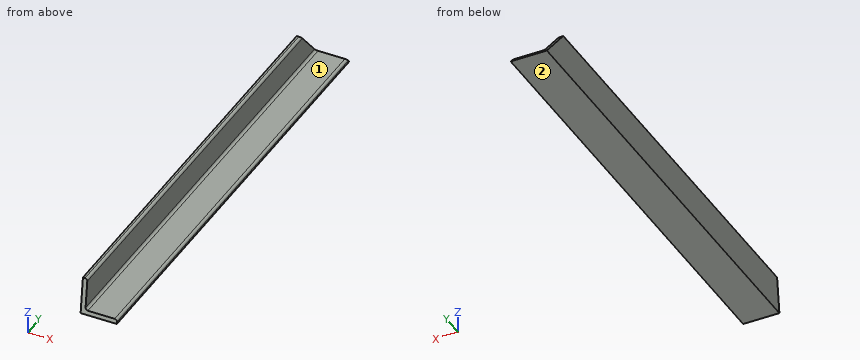
from build123d import *

# Parameters (mm, degrees)
F1_DEPTH = 474.6625
F2_R     = 5.08
F4_DEPTH = 76.2
F5_DEPTH = 76.2


with BuildPart() as f1:
    # F0 (on Front) → F1 (new body, symmetric)
    with BuildSketch(Plane.XZ):
        Polygon((0, 76.2), (0, 0), (76.2, 0), (76.2, 9.525), (9.525, 9.525), (9.525, 76.2), align=None)
    extrude(amount=F1_DEPTH, both=True)

    # F2
    f2_edges = [f1.edges().sort_by_distance(p)[0] for p in [
        (9.525, 0, 76.2),
        (9.525, 0, 9.525),
        (76.2, 0, 9.525),
    ]]
    fillet(f2_edges, radius=F2_R)

    # F3 (on face) → F4 (cut)
    with BuildSketch(Plane(origin=(0, 0, 0), x_dir=(0, -1, 0), z_dir=(-1, 0, 0))):
        Polygon((-474.6625, 76.2), (-474.6625, 0), (-407.483163, 76.2), align=None)
        Polygon((465.306316, 76.2), (474.6625, 0), (474.6625, 76.2), align=None)
    extrude(amount=-F4_DEPTH, mode=Mode.SUBTRACT)

    # F3 (on face) → F5 (cut)
    with BuildSketch(Plane(origin=(0, 0, 0), x_dir=(0, -1, 0), z_dir=(-1, 0, 0))):
        Polygon((-474.6625, 76.2), (-474.6625, 0), (-407.483163, 76.2), align=None)
        Polygon((465.306316, 76.2), (474.6625, 0), (474.6625, 76.2), align=None)
    extrude(amount=-F5_DEPTH, mode=Mode.SUBTRACT)


solid = f1.part
Check sheet for the modelled part. Datum: model origin and axes. Units: mm. Face numbers are marked on the shaded views. A direction names the side the tool comes from. Round coordinates to 2 decimals unless told otherwise and drop trailing zeros. Order: outer loops, then holes, each group sorted by start corner. A loop starts at its lowest first (then second) coordinate and runs counter-clockwise, first axis right, second up.
(1) Access from +Z, -Z, +X, -X, +Y, -Y to the whole of each face (thin tool, end or side, straight path). Record for the marked faces 1 and 2.
(2) Go/stop test with flat-tipped pins: P1, Ø2, axis at y = 212.5, z = 18, coming from the +X side (3 decimals); P2, Ø8, axis at x = 16.5, y = 344, coming from the +Z side; P3, Ø6, axis at y = 170, z = 10, coming from the +X side. Record where each tip stops, or that it passes through.
(3) Scan lines: probe 1 along X at (y, z) = (45, 67) (3 decimals); probe 2 along X at (y, z) = (-142, 5.5). Record each from-to range of solid material in increasing order.
(4) Cross-section at C-C, the plane z = 37. Enter the section's corners in (x, y) (3 decimals), and give its area (3 significant figures).
(5) Cross-section at B-B, the plane x = 24. Enter the section's corners in (y, z) (1 decimal).
(6) Cross-section at A-A, the plane y = -128. Enter the section's corners in (x, z) (3 decimals).
Check sheet entries:
1. face 1: +Z, +X, +Y, -Y
1. face 2: -Z, +X, -X, +Y, -Y
2. P1: stops at x = 9.525
2. P2: stops at z = 9.98
2. P3: stops at x = 75.51
3. probe 1: x = 0 to 9.525
3. probe 2: x = 0 to 76.09
4. outline: (0, -470.119) - (9.525, -470.119) - (9.525, 442.043) - (0, 442.043) - close
4. area: 8,690 mm2
5. outline: (-474.7, 0) - (474.7, 0) - (466.3, 9.5) - (-473.5, 9.5) - close
6. outline: (0, 0) - (76.2, 0) - (76.2, 4.445) arc R5.08 ccw to (71.12, 9.525) - (14.605, 9.525) arc R5.08 cw to (9.525, 14.605) - (9.525, 71.12) arc R5.08 ccw to (4.445, 76.2) - (0, 76.2) - close
